Design review of the part built by this model. Coordinates are the model's own, in mm. A direction names the side the tool comes from. Give positions to 0.01 mm unless a question says otherwise; leave off trailing zeros. Loops run counter-clockwise (first coordinate to the right, second up) from the corner with the lowest first, then second, coordinate; pieces in that order, holes last. Notation, with made-up numbers: (45, 1.5) -> (89, 1.5) arc R33 cw to (89, 36.5) -> close; hole circle Ø1 at (40, 43.5). An arc over 180 degrees is marked (long way). Use a Markdown table: item, result. Add a question column.
1. For pin 1 Ø3 at (x, y) = (9, 0.5) entering from +Z; pin 2 Ø0.9 at (x, y) = (6, 1.5) entering from -Z; pin 3 Ø0.9 at (x, z) = (3, -33) entering from -Y; pin 4 Ø5.5 at (x, z) = (7, -9.5) entering from -Y, all flat-tipped, find the tip position at first contact; note any pin that passes through.
2. For faces 1 (the flat face through (7, 2, -17.5)), 2 (the flat face through (7, 3, -10)), 3 (the flat face through (3, 3, -31)), list the 3-axis set-ups (+Z, -Z, +X, -X, +Y, -Y) from which the entire face can be reached by the end or side of a thin tool; tool diameter is ignored.
3. Add section A-A (z = -4). State the section outline as (x, y) points.
4. Add section B-B (y = 2.65). State the section outline as (x, z) points.
5. Add section C-C (x = 9). State the section outline as (y, z) points.
6. Draft analysis for pull direction Z (two halves, no side actions). For faces 4 (the flat face through (15, 2, -17)), 5 (the flat face through (7, 1, -6.5)), 6 (the cylindrical face through (2, 2, -16)), 7 (the flat face through (9, 3, -34)), state which applies: pulls with the +Z half, pulls with the -Z half, needs draft (parallel to the pull), parting line crosses it, or undercut.
7. Add section D-D (x = 1.5). State the section outline as (y, z) points.
8. To check wall thickness, follow line 1 (Z direction, x = 7.25, y = 1.9); line 2 (Z direction, x = 3.5, y = 0.8); line 3 (Z direction, x = 11.5, y = 3.45). State the ranges of each line that lie inside material, in increasing order.
```python
from build123d import *

# Parameters (mm, degrees)
EXTRUDE_1_DEPTH     = 5
SKETCH_2_W          = 7
SKETCH_2_H          = 3
CUT_EXTRUDE_1_DEPTH = 16
SKETCH_3_W          = 3
SKETCH_3_H          = 2
CUT_EXTRUDE_2_DEPTH = 12


with BuildPart() as part:
    # 草图1 → 凸台-拉伸1 (new body)
    with BuildSketch(Plane(origin=(0, 0, 0), x_dir=(1, 0, 0), z_dir=(0, 1, 0))):
        Polygon((15, 34), (0, 34), (0, 31), (7, 31), (7, 26), (0, 26), (0, 0), (15, 0), align=None)
        with BuildLine():
            ThreePointArc((3.5, 2.5), (2, 4), (3.5, 5.5))
            Line((3.5, 5.5), (11.5, 5.5))
            ThreePointArc((11.5, 5.5), (13, 4), (11.5, 2.5))
            Line((11.5, 2.5), (3.5, 2.5))
        make_face(mode=Mode.SUBTRACT)
        with BuildLine():
            ThreePointArc((3.5, 14.5), (2, 16), (3.5, 17.5))
            Line((3.5, 17.5), (11.5, 17.5))
            ThreePointArc((11.5, 17.5), (13, 16), (11.5, 14.5))
            Line((11.5, 14.5), (3.5, 14.5))
        make_face(mode=Mode.SUBTRACT)
    extrude(amount=EXTRUDE_1_DEPTH)

    # 草图2 → 切除-拉伸1 (cut, through all)
    with BuildSketch(Plane.ZY):
        with Locations((-10, 1.5)):
            Rectangle(SKETCH_2_W, SKETCH_2_H)
    extrude(amount=-CUT_EXTRUDE_1_DEPTH, mode=Mode.SUBTRACT)

    # 草图3 → 切除-拉伸2 (cut)
    with BuildSketch(Plane.ZY.offset(-7)):
        with Locations((-32.5, 1)):
            Rectangle(SKETCH_3_W, SKETCH_3_H)
    extrude(amount=CUT_EXTRUDE_2_DEPTH, mode=Mode.SUBTRACT)


solid = part.part
```
Taken from the geometry:
| question | item | result |
|---|---|---|
| 1 | pin 1 | stops at z = 0 |
| 1 | pin 2 | stops at z = -26 |
| 1 | pin 3 | stops at y = 2 |
| 1 | pin 4 | stops at y = 3 |
| 2 | face 1 | +Y, -Y |
| 2 | face 2 | +X, -X, -Y |
| 2 | face 3 | -X, +Y, -Y |
| 3 | outline | (0, 0) -> (2, 0) -> (2, 5) -> (0, 5) -> close; (13, 0) -> (15, 0) -> (15, 5) -> (13, 5) -> close |
| 4 | outline | (0, -34) -> (15, -34) -> (15, -13.5) -> (0, -13.5) -> (0, -26) -> (7, -26) -> (7, -31) -> (0, -31) -> close; (0, -6.5) -> (15, -6.5) -> (15, 0) -> (0, 0) -> close; hole (3.5, -17.5) -> (11.5, -17.5) arc R1.5 ccw to (11.5, -14.5) -> (3.5, -14.5) arc R1.5 ccw to start; hole (3.5, -5.5) -> (11.5, -5.5) arc R1.5 ccw to (11.5, -2.5) -> (3.5, -2.5) arc R1.5 ccw to start |
| 5 | outline | (0, -34) -> (5, -34) -> (5, -17.5) -> (0, -17.5) -> close; (0, -14.5) -> (5, -14.5) -> (5, -5.5) -> (0, -5.5) -> (0, -6.5) -> (3, -6.5) -> (3, -13.5) -> (0, -13.5) -> close; (0, -2.5) -> (5, -2.5) -> (5, 0) -> (0, 0) -> close |
| 6 | face 4 | needs draft |
| 6 | face 5 | undercut |
| 6 | face 6 | undercut |
| 6 | face 7 | pulls with the -Z half |
| 7 | outline | (0, -26) -> (5, -26) -> (5, 0) -> (0, 0) -> (0, -6.5) -> (3, -6.5) -> (3, -13.5) -> (0, -13.5) -> close; (2, -34) -> (5, -34) -> (5, -31) -> (2, -31) -> close |
| 8 | line 1 | z = -34 to -17.5, -14.5 to -13.5, -6.5 to -5.5, -2.5 to 0 |
| 8 | line 2 | z = -26 to -17.5, -14.5 to -13.5, -6.5 to -5.5, -2.5 to 0 |
| 8 | line 3 | z = -34 to -17.5, -14.5 to -5.5, -2.5 to 0 |
